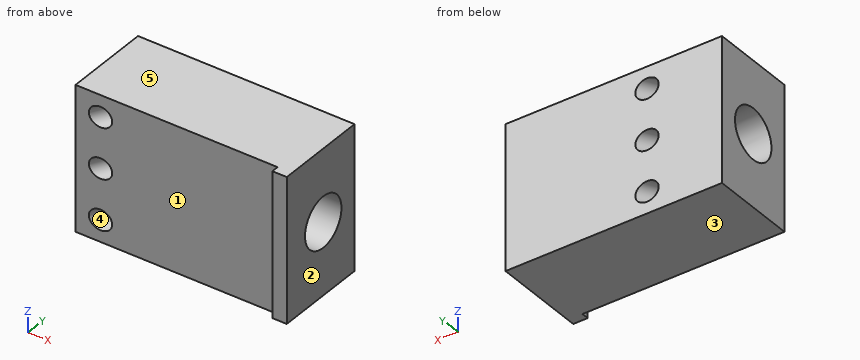
```python
from build123d import *

# Parameters (mm, degrees)
SKICA1_W                 = 30
SKICA1_H                 = 12
SKICA1_W_2               = 2
SKICA1_H_2               = 1
P_IDAT_VYSUNUT_M1_DEPTH  = 20
SKICA2_R                 = 3.5
ODEBRAT_VYSUNUT_M1_DEPTH = 34
SKICA3_R                 = 1.4
ODEBRAT_VYSUNUT_M2_DEPTH = 34


with BuildPart() as part:
    # Skica1 → Přidat vysunutím1 (new body)
    with BuildSketch(Plane.XY):
        with Locations((15, 6)):
            Rectangle(SKICA1_W, SKICA1_H)
        with Locations((29, -0.5)):
            Rectangle(SKICA1_W_2, SKICA1_H_2)
    extrude(amount=P_IDAT_VYSUNUT_M1_DEPTH)

    # Skica2 → Odebrat vysunutím1 (cut)
    with BuildSketch(Plane.ZY):
        with Locations((10, 6)):
            Circle(SKICA2_R)
    extrude(amount=-ODEBRAT_VYSUNUT_M1_DEPTH, mode=Mode.SUBTRACT)

    # Skica3 → Odebrat vysunutím2 (cut)
    with BuildSketch(Plane(origin=(0, 0, 0), x_dir=(0, 0, -1), z_dir=(-0.500000000000001, -0.866025403784438, 0))):
        with Locations(Location((-10, 3, 0), (0, 0, 90))):
            Circle(SKICA3_R)
        with Locations(Location((-17, 3, 0), (0, 0, 270))):
            Circle(SKICA3_R)
        with Locations(Location((-3, 3, 0), (0, 0, 270))):
            Circle(SKICA3_R)
    extrude(amount=-ODEBRAT_VYSUNUT_M2_DEPTH, mode=Mode.SUBTRACT)


solid = part.part
```
Work out the finished part from the listing and answer in its coordinate system (mm). Face numbers are marked on the shaded views. A direction names the side the tool comes from. Round coordinates to 2 decimals unless told otherwise and drop trailing zeros. Order: outer loops, then holes, each group sorted by start corner. A loop starts at its lowest first (then second) coordinate and runs counter-clockwise, first axis right, second up.
Q1. Given pin 1 Ø12 at (x, z) = (8.5, 8.5) entering from -Y, flat-ended and moving along its own axis, determine where the tip first touches the part or whether it passes through.
Solution:
pin 1: stops at y = 0
Q2. A tool of negligible diameter and unlimited length cuts with its end or side. For the marked faces 1 and 2, from which of +Z, -Z, +X, -X, +Y, -Y can it reach the whole face along a straight path? Write none if from no direction.
Solution:
face 1: +Z, -Z, -X, -Y
face 2: +Z, -Z, +X, +Y, -Y
Q3. The mould has two halves that part along Z. Classify the marked faces 3, 4 and 5: pulls with the +Z half, pulls with the -Z half, needs draft (parallel to the pull), parting line crosses it, or undercut.
Solution:
face 3: pulls with the -Z half
face 4: undercut
face 5: pulls with the +Z half
Q4. A cutting plane is placed at B-B, the plane z = 16.25. Determine the outline of the cut face in (x, y).
Solution:
outline: (0, 0) - (2.1, 0) - (9.03, 12) - (0, 12) - close; (4.83, 0) - (28, 0) - (28, -1) - (30, -1) - (30, 12) - (11.76, 12) - close
Q5. A cutting plane is placed at C-C, the plane y = 6. Count the separate pieces of the cut face and the enclosed holes in it, then the cut area to 3 significant figures.
Solution:
separate pieces: 2
enclosed holes: 2
area: 376 mm2
Q6. Find the intervals of material crossed by line 1 along Y through (x, z) = (24, 10); line 2 along Z through (x, y) = (11, 11.25); line 3 along Z through (x, y) = (3, 0.25), in increasing order.
Solution:
line 1: y = 0 to 2.5, 9.5 to 12
line 2: z = 0 to 1.93, 4.07 to 8.93, 11.07 to 15.93, 18.07 to 20
line 3: z = 0 to 1.7, 4.3 to 8.7, 11.3 to 15.7, 18.3 to 20
Q7. A cutting plane is placed at A-A, the plane x = 26. Determine the outline of the cut face in (y, z), then the cut area to 3 significant figures.
Solution:
outline: (0, 0) - (12, 0) - (12, 20) - (0, 20) - close; hole circle Ø7 at (6, 10)
area: 202 mm2
Q8. A cutting plane is placed at D-D, the plane z = 14. Determine the outline of the cut face in (x, y).
Solution:
outline: (0, 0) - (28, 0) - (28, -1) - (30, -1) - (30, 12) - (0, 12) - close
